Check sheet for the drawn part. Datum: minimum x, y, z corner. Units: mm. Give positions to 0.01 mm unless a question says otherwise; leave off trailing zeros. Order: outer loops, then holes, each group sorted by start corner. A loop starts at its lowest first (then second) coordinate and runs counter-clockwise, first axis right, second up. Notation, with made-up numbers: (27, 54.5) - (42, 54.5) arc R16 ccw to (42, 80.5) - close; hole circle Ø2 at (77.5, -21.75). An arc over 180 degrees is marked (long way). Answer as a JSON object with one key per item and string values. Group by question number.
(1) Section check D-D (z = 12). Record the boundary of the cut face in (x, y), then the cut area to 3 significant figures.
(2) Section check A-A (z = 16). Record the boundary of the cut face in (x, y), then the cut area to 3 significant figures.
(3) Thickness scan on line 1 (Z direction, x = 12.5, y = 0.95); line 2 (Z direction, x = 13.5, y = 2.6); line 3 (Z direction, x = 20.5, y = 2.1). Record the ranges inside material, lowest first.
(4) Section check C-C (x = 4.5). Record the boundary of the cut face in (y, z), then the cut area to 3 significant figures.
(5) Section check B-B (y = 2.3). Record the boundary of the cut face in (x, z), then the cut area to 3 significant figures.
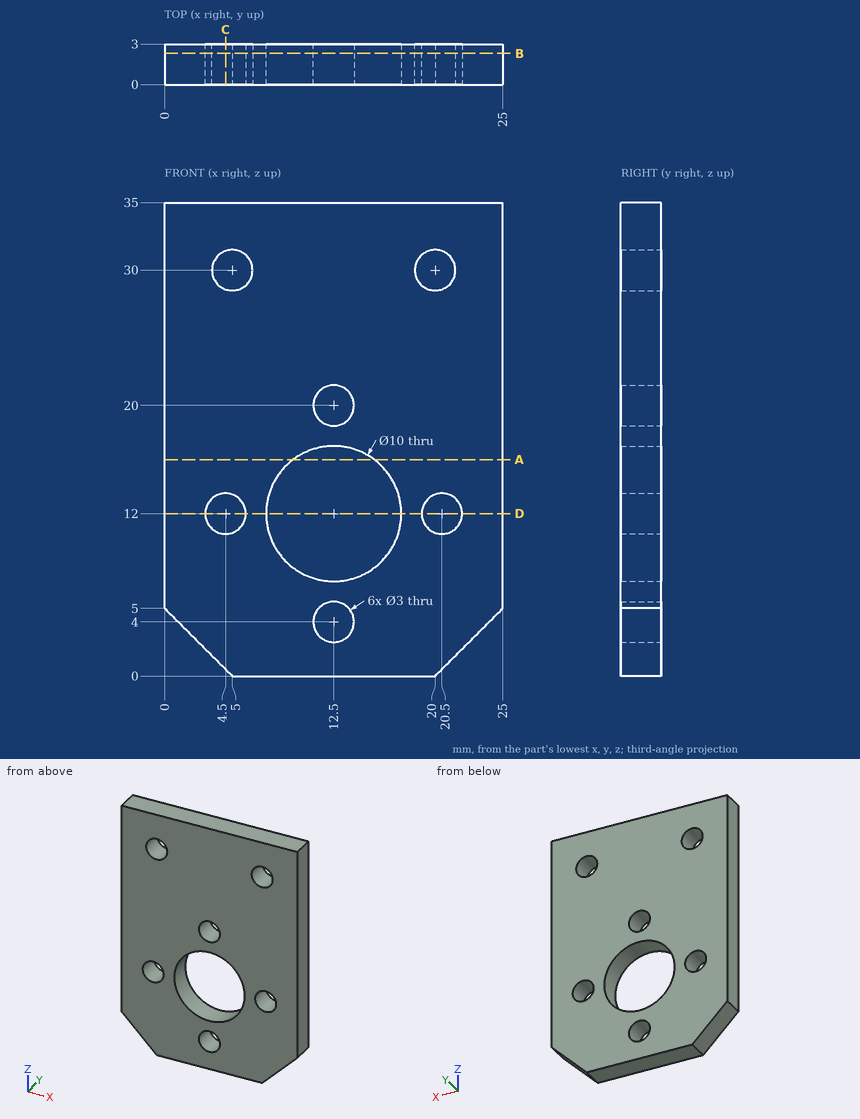
Solutions:
{
 "1": {"outline": "(0, 0) - (3, 0) - (3, 3) - (0, 3) - close; (6, 0) - (7.5, 0) - (7.5, 3) - (6, 3) - close; (17.5, 0) - (19, 0) - (19, 3) - (17.5, 3) - close; (22, 0) - (25, 0) - (25, 3) - (22, 3) - close", "area": "27.0 mm2"},
 "2": {"outline": "(0, 0) - (9.5, 0) - (9.5, 3) - (0, 3) - close; (15.5, 0) - (25, 0) - (25, 3) - (15.5, 3) - close", "area": "57.0 mm2"},
 "3": {"line 1": "z = 0 to 2.5, 5.5 to 7, 17 to 18.5, 21.5 to 35", "line 2": "z = 0 to 2.88, 5.12 to 7.1, 16.9 to 18.88, 21.12 to 35", "line 3": "z = 0.5 to 10.5, 13.5 to 28.59, 31.41 to 35"},
 "4": {"outline": "(0, 0.5) - (3, 0.5) - (3, 10.5) - (0, 10.5) - close; (0, 13.5) - (3, 13.5) - (3, 28.59) - (0, 28.59) - close; (0, 31.41) - (3, 31.41) - (3, 35) - (0, 35) - close", "area": "86.0 mm2"},
 "5": {"outline": "(0, 5) - (5, 0) - (20, 0) - (25, 5) - (25, 35) - (0, 35) - close; hole circle Ø3 at (4.5, 12); hole circle Ø3 at (5, 30); hole circle Ø10 at (12.5, 12); hole circle Ø3 at (12.5, 4); hole circle Ø3 at (12.5, 20); hole circle Ø3 at (20, 30); hole circle Ø3 at (20.5, 12)", "area": "729 mm2"}
}
